Here's how the part is built. I have some questions about the finished solid (model axes, mm). Coordinates: 2 decimals unless noted, no trailing zeros. Loops run counter-clockwise (first coordinate to the right, second up) from the corner with the lowest first, then second, coordinate; pieces in that order, holes last. Notation, with made-up numbers: (24.5, 47.25) -> (74.5, 47.25) arc R20 ccw to (74.5, 79.25) -> close; hole circle Ø4 at (-3.5, 35.5). An arc over 180 degrees is marked (long way). Answer as a JSON object with one key per item and string values. Group by question number.
1) I want a section at D-D (x = -35.04). Write out the boundary of the cut face in (y, z) (3 decimals).
2) I want a section at B-B (y = 2.75). Write out the boundary of the cut face in (x, z) (3 decimals), then the cut area to 3 significant figures.
3) I want a section at A-A (x = 35.04). Write out the boundary of the cut face in (y, z) (3 decimals), then the cut area to 3 significant figures.
4) If we mould it in two halves opening along Y, with no side actions, what happens to faces 1 (the cylindrical face through (-8.647, 0.167, 6.454)), 2 (the flat face through (-1, 6.35, 6)), 3 (the cylindrical face through (-17.942, -0.089, 6.273))? For each: +Y half, -Y half, draft (parallel to the pull), parting line (faces both ways), or undercut.
5) I need wall thicknesses on probe 1 along X at (y, z) = (4, 2.25); probe 2 along X at (y, z) = (2.75, 6); probe 3 along Z at (x, y) = (-35.04, 3.75) (3 decimals). Which ranges of each line are inside material? Lowest first, please. Write a range as [from, to].
6) I want a section at C-C (z = 7.25). Write out the boundary of the cut face in (x, y).
```python
from build123d import *

# Parameters (mm, degrees)
SKETCH1_W             = 80.08
SKETCH1_H             = 12.7
BOSS_EXTRUDE1_DEPTH   = 12.73
M5X0_8_TAPPED_HOLE1_D = 4.2
M4X0_7_TAPPED_HOLE1_D = 3.3
SKETCH7_R             = 5.21
CUT_EXTRUDE1_DEPTH    = 12.73


with BuildPart() as part:
    # Sketch1 → Boss-Extrude1 (new body)
    with BuildSketch(Plane.XY):
        Rectangle(SKETCH1_W, SKETCH1_H)
    extrude(amount=BOSS_EXTRUDE1_DEPTH)

    # M5x0.8 Tapped Hole1 (through all)
    with Locations(Plane(origin=(0, 6.35, 0), x_dir=(1, 0, 0), z_dir=(0, 1, 0))):
        with Locations((-35.04, -6.365), (-20.04, -6.365)):
            Hole(M5X0_8_TAPPED_HOLE1_D / 2)

    # M4x0.7 Tapped Hole1 (through all)
    with Locations(Plane(origin=(0, 6.35, 0), x_dir=(1, 0, 0), z_dir=(0, 1, 0))):
        with Locations((20.04, -6.365), (35.04, -6.365)):
            Hole(M4X0_7_TAPPED_HOLE1_D / 2)

    # Sketch7 → Cut-Extrude1 (cut)
    with BuildSketch(Plane.XY.offset(12.73)):
        with Locations((3.44, 0)):
            Circle(SKETCH7_R)
        with Locations((-3.44, 0)):
            Circle(SKETCH7_R)
    extrude(amount=-CUT_EXTRUDE1_DEPTH, mode=Mode.SUBTRACT)


solid = part.part
```
Determined:
{
 "1": {"outline": "(-6.35, 0) -> (6.35, 0) -> (6.35, 4.265) -> (-6.35, 4.265) -> close; (-6.35, 8.465) -> (6.35, 8.465) -> (6.35, 12.73) -> (-6.35, 12.73) -> close"},
 "2": {"outline": "(-40.04, 0) -> (-7.865, 0) -> (-7.865, 12.73) -> (-40.04, 12.73) -> close; (7.865, 0) -> (40.04, 0) -> (40.04, 12.73) -> (7.865, 12.73) -> close; hole circle Ø4.2 at (-35.04, 6.365); hole circle Ø4.2 at (-20.04, 6.365); hole circle Ø3.3 at (20.04, 6.365); hole circle Ø3.3 at (35.04, 6.365)", "area": "774 mm^2"},
 "3": {"outline": "(-6.35, 0) -> (6.35, 0) -> (6.35, 4.715) -> (-6.35, 4.715) -> close; (-6.35, 8.015) -> (6.35, 8.015) -> (6.35, 12.73) -> (-6.35, 12.73) -> close", "area": "120 mm^2"},
 "4": {"face 1": "undercut", "face 2": "+Y half", "face 3": "draft"},
 "5": {"probe 1": "[-40.04, -6.78], [-0.1, 0.1], [6.78, 40.04]", "probe 2": "[-40.04, -37.11], [-32.97, -22.11], [-17.97, -7.87], [7.87, 18.43], [21.65, 33.43], [36.65, 40.04]", "probe 3": "[0, 4.265], [8.465, 12.73]"},
 "6": {"outline": "(-40.04, -6.35) -> (-36.94, -6.35) -> (-36.94, 6.35) -> (-40.04, 6.35) -> close; (-33.14, -6.35) -> (-21.94, -6.35) -> (-21.94, 6.35) -> (-33.14, 6.35) -> close; (-18.14, -6.35) -> (18.65, -6.35) -> (18.65, 6.35) -> (-18.14, 6.35) -> close; (21.43, -6.35) -> (33.65, -6.35) -> (33.65, 6.35) -> (21.43, 6.35) -> close; (36.43, -6.35) -> (40.04, -6.35) -> (40.04, 6.35) -> (36.43, 6.35) -> close; hole (0, -3.91) arc R5.21 ccw (long way) to (0, 3.91) arc R5.21 ccw (long way) to start"}
}
